Geometry: see drawing. Coordinates: mm, zero at the bounding-box minimum. Coordinates: 2 decimals unless noted, no trailing zeros. Write each loop counter-clockwise with the first axis right and the second up, starting at its lowest first coordinate (ties: lowest second). Pieces come first, ordered by that corner, then holes. Notation, with made-up numbers: M 21,51.5 L 49,51.5 A32 ccw 49,82.5 Z; hole C 43.5,71 d3. An arc over 180 degrees is marked long. Answer as CSV lines item,"result". Start each with the question number.
1. Section C-C on z = 7.5. Return the cut outline in (x, y).
2. Contact query for flat-ended pins moving along their axis: pin 1 Ø1.5 at (y, z) = (22.5, 3) entering from +X; pin 2 Ø14.5 at (x, y) = (14, 10) entering from -Z; pin 3 Ø3 at (x, z) = (20, 9) entering from -Y. Output: stop coordinate, or through.
3. Section D-D on z = 18. Return the cut outline in (x, y).
4. Mould query, pull axis X, two halves, no side actions, for the marked faces 1, 2 and 3. Classes: pulls with the +X half, pulls with the -X half, needs draft (parallel to the pull), parting line crosses it, or undercut.
5. Section A-A on x = 13. Return the cut outline in (y, z), plus the area to 3 significant figures.
6. Line query: probe 1 along Y at (x, z) = (13, 8.75); probe 2 along Z at (x, y) = (10.5, 13); probe 3 along Y at (x, z) = (23, 14.5). Output: solid intervals per line, ascending. Write a range as [from, to].
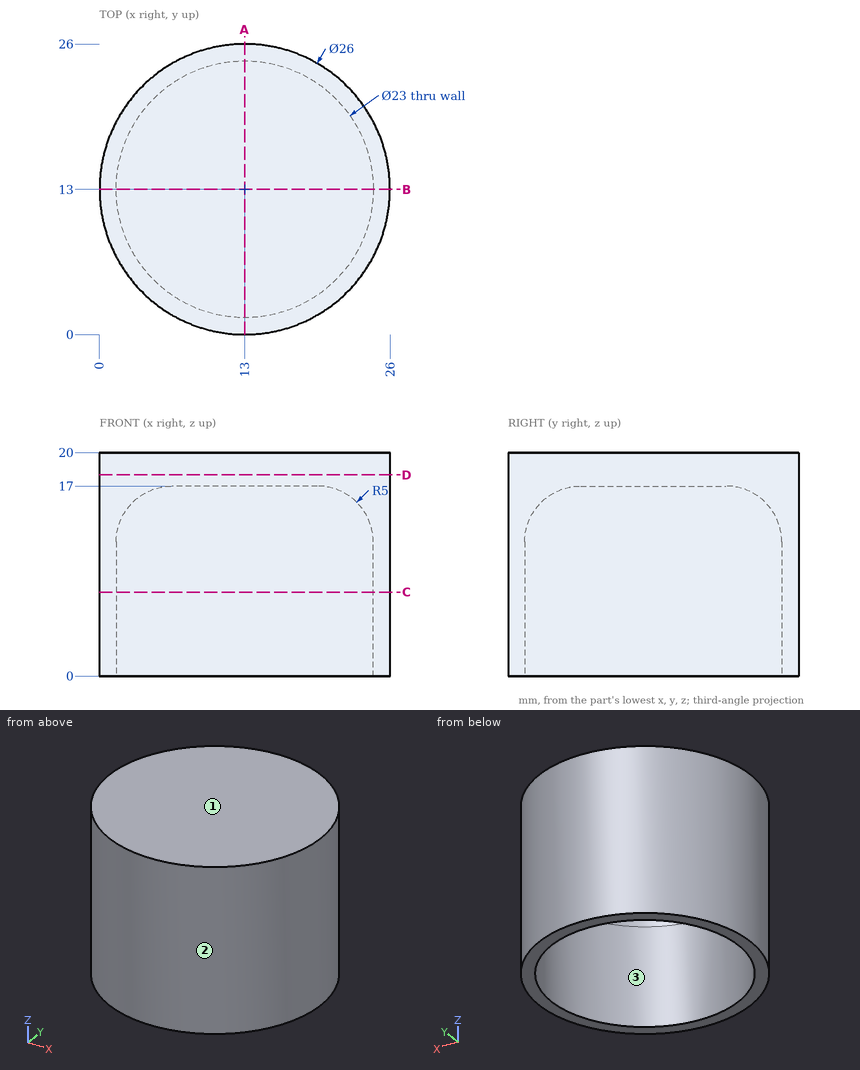
Values:
1,outline,"C 13,13 d26; hole C 13,13 d23"
2,pin 1,"x = 22.61"
2,pin 2,"z = 15.11"
2,pin 3,"y = 1.22"
3,outline,"C 13,13 d26"
4,face 1,"needs draft"
4,face 2,"parting line crosses it"
4,face 3,"undercut"
5,outline,"M 0,0 L 1.5,0 L 1.5,12 A5 cw 6.5,17 L 19.5,17 A5 cw 24.5,12 L 24.5,0 L 26,0 L 26,20 L 0,20 Z"
5,area,"140 mm²"
6,probe 1,"[0, 1.5], [24.5, 26]"
6,probe 2,"[17, 20]"
6,probe 3,"[4.69, 8.84], [17.16, 21.31]"
